from build123d import *

# Parameters (mm, degrees)
F0_W            = 50
F0_H            = 150
F0_H_2          = 50
F0_W_2          = 60
F0_W_3          = 70
F0_H_3          = 35
F1_DEPTH        = 10
F2_W            = 10
F2_H            = 50
F3_DEPTH        = 30
F4_R            = 5.5
F5_DEPTH        = 190.001
F6_R            = 3.175
F7_DEPTH        = 10.001
F8_R            = 5.5
F9_DEPTH        = 10.001
F10_R           = 5.5
F11_DEPTH       = 10.001
F13_DEPTH       = 10.001
F14_W           = 6
F14_H           = 30
F15_DEPTH       = 32
F16_R           = 5.5
F17_DEPTH       = 76.001
F19_D           = 3.1
F19_CSINK_D     = 5.6
F19_CSINK_ANGLE = 90
F21_D           = 2
F21_DEPTH       = 30
F21_TIP         = 0.600860619


with BuildPart() as f1:
    # F0 (on Top) → F1 (new body)
    with BuildSketch(Plane.XY):
        Rectangle(F0_W, F0_H)
        with Locations((0, 100)):
            Rectangle(F0_W, F0_H_2)
        with Locations((55, 100)):
            Rectangle(F0_W_2, F0_H_2)
        with Locations((-55, 100)):
            Rectangle(F0_W_2, F0_H_2)
        with Locations((0, -100)):
            Rectangle(F0_W, F0_H_2)
        with Locations((60, -100)):
            Rectangle(F0_W_3, F0_H_2)
        with Locations((0, 142.5)):
            Rectangle(F0_W, F0_H_3)
        with Locations((-60, -100)):
            Rectangle(F0_W_3, F0_H_2)
    extrude(amount=F1_DEPTH)

    # F2 (on face) → F3 (join)
    with BuildSketch(Plane.XY.offset(10)):
        with Locations((-90, -100)):
            Rectangle(F2_W, F2_H)
        with Locations((90, -100)):
            Rectangle(F2_W, F2_H)
    extrude(amount=F3_DEPTH)

    # F4 (on face) → F5 (cut, through all)
    with BuildSketch(Plane(origin=(-95, 0, 0), x_dir=(0, -1, 0), z_dir=(-1, 0, 0))):
        with Locations((100, 30.5)):
            Circle(F4_R)
    extrude(amount=-F5_DEPTH, mode=Mode.SUBTRACT)

    # F6 (on face) → F7 (cut, through all)
    with BuildSketch(Plane.XY.offset(10)):
        with Locations((0, 152.825)):
            Circle(F6_R)
    extrude(amount=-F7_DEPTH, mode=Mode.SUBTRACT)

    # F8 (on face) → F9 (cut, through all)
    with BuildSketch(Plane.XY.offset(10)):
        with Locations((-69.5, 100)):
            Circle(F8_R)
    extrude(amount=-F9_DEPTH, mode=Mode.SUBTRACT)

    # F10 (on face) → F11 (cut, through all)
    with BuildSketch(Plane.XY.offset(10)):
        with Locations((69.5, 100)):
            Circle(F10_R)
    extrude(amount=-F11_DEPTH, mode=Mode.SUBTRACT)

    # F12 (on face) → F13 (cut, through all)
    with BuildSketch(Plane.XY.offset(10)):
        with BuildLine():
            Line((17.7911710483, 82.2515942001), (27.4237727452, 85))
            ThreePointArc((27.4237727452, 85), (24.83, 100), (27.4237727452, 115))
            Line((27.4237727452, 115), (17.7911710483, 117.7484057999))
            ThreePointArc((17.7911710483, 117.7484057999), (14.83, 100), (17.7911710483, 82.2515942001))
        make_face()
        with BuildLine():
            Line((-27.4237727452, 85), (-17.7911710483, 82.2515942001))
            ThreePointArc((-17.7911710483, 82.2515942001), (-14.83, 100), (-17.7911710483, 117.7484057999))
            Line((-17.7911710483, 117.7484057999), (-27.4237727452, 115))
            ThreePointArc((-27.4237727452, 115), (-24.83, 100), (-27.4237727452, 85))
        make_face()
    extrude(amount=-F13_DEPTH, mode=Mode.SUBTRACT)

    # F14 (on face) → F15 (join)
    with BuildSketch(Plane.XY.offset(10)):
        with Locations((22, 6.836565081)):
            Rectangle(F14_W, F14_H)
    extrude(amount=F15_DEPTH)

    # F16 (on face) → F17 (cut, through all)
    with BuildSketch(Plane(origin=(19, 0, 0), x_dir=(0, -1, 0), z_dir=(-1, 0, 0))):
        with Locations((-6.426565081, 30.5)):
            Circle(F16_R)
    extrude(amount=-F17_DEPTH, mode=Mode.SUBTRACT)

    # F19 (through all)
    with Locations(Plane.YZ.offset(25)):
        with Locations((6.426565081, 38.4), (14.326565081, 30.5), (6.426565081, 22.6), (-1.473434919, 30.5)):
            CounterSinkHole(F19_D / 2, F19_CSINK_D / 2, counter_sink_angle=F19_CSINK_ANGLE)

    # F21
    with Locations(Plane.YZ.offset(95)):
        with Locations((-107.1, 30.5), (-92.9, 30.5), (-91.0878232998, 21.4521767002), (-109.0478232998, 21.5878232998)):
            Hole(F21_D / 2, depth=F21_DEPTH)
            with Locations((0, 0, -(F21_DEPTH + F21_TIP / 2))):  # 118° drill point
                Cone(0, F21_D / 2, F21_TIP, mode=Mode.SUBTRACT)


solid = f1.part
For this review, take the finished solid that the model builds, in its own axes (mm). A direction names the side the tool comes from. Give positions to 0.01 mm unless a question says otherwise; leave off trailing zeros. Loops run counter-clockwise (first coordinate to the right, second up) from the corner with the lowest first, then second, coordinate; pieces in that order, holes last. Notation, with made-up numbers: M 43.5,88 L 90.5,88 A9 ccw 90.5,102 Z; hole C 89,-10.5 d5. An arc over 180 degrees is marked long. Answer as a JSON object with one key per item and string values. Group by question number.
Q1. For probe 1 along Y at (x, z) = (20.15, 30.5); probe 2 along Y at (x, z) = (-69.5, 5); probe 3 along Y at (x, z) = (0, 6.5), list the stretches that pass through material, from the lowest coordinate up. Write a range as [from, to].
Q2. Mouldability with a two-part tool opening along Y and no side actions: class faces 1 (the cylindrical face through (-90.07, -94.505, 30.742)), 2 (the flat face through (22, -8.163, 26)), 3 (the flat face through (22, 7, 42)), 4 (the cylindrical face through (-14.83, 99.75, 5.07)) as +Y half, -Y half, draft (parallel to the pull), parting line (faces both ways), or undercut.
Q3. Add section D-D on y = 100. Give the boundary of the cut face in (x, z).
Q4. Insertion check: P1, Ø3, axis at x = 23, z = 21, coming from the +Y side; P2, Ø10, axis at x = 0.5, y = -67, coming from the +Z side; P3, Ø6.5, axis at y = 6.43, z = 30.5, coming from the -X side; P4, Ø4, axis at y = 21, z = 8.5, coming from the +X side. Each pin has a flat end and moves straight along its axis. Give the tip position at first contact, or say it passes through.
Q5. Tool access review of faces 5 (the flat face through (-67.9, -75, 9.5)), 6 (the flat face through (-85, -100.4, 24.8)), 7 (the flat face through (70, -75, 8)), 8 (the cylindrical face through (14.83, 100.25, 5.07)), 9 (the flat face through (55, 125, 5)): name each direction out of +Z, -Z, +X, -X, +Y, -Y from which nothing blocks a thin tool from reaching the whole face with its end or side.
Q6. Add section C-C on z = 16. Give the boundary of the cut face in (x, y).
Q7. Add section B-B on y = -100. Give the boundary of the cut face in (x, z).
Q8. Add section A-A on x = 0. Give the boundary of the cut face in (y, z).
Checked values:
{
 "1": {"probe 1": "[-8.16, -3.02], [0.08, 0.93], [11.93, 12.78], [15.88, 21.84]", "probe 2": "[-125, -75], [75, 94.5], [105.5, 125]", "probe 3": "[-125, 149.65], [156, 160]"},
 "2": {"face 1": "undercut", "face 2": "-Y half", "face 3": "draft", "face 4": "undercut"},
 "3": {"outline": "M -85,0 L -75,0 L -75,10 L -85,10 Z; M -64,0 L -24.83,0 L -24.83,10 L -64,10 Z; M -14.83,0 L 14.83,0 L 14.83,10 L -14.83,10 Z; M 24.83,0 L 64,0 L 64,10 L 24.83,10 Z; M 75,0 L 85,0 L 85,10 L 75,10 Z"},
 "4": {"P1": "y = 21.84", "P2": "z = 10", "P3": "through", "P4": "x = 25"},
 "5": {"face 5": "+Z, -Z, -X", "face 6": "+Z, +Y, -Y", "face 7": "+Z, -Z, +X", "face 8": "+Z, -Z", "face 9": "+Z, -Z, +X, +Y"},
 "6": {"outline": "M -95,-125 L -85,-125 L -85,-75 L -95,-75 Z; M 19,-8.16 L 25,-8.16 L 25,21.84 L 19,21.84 Z; M 85,-125 L 95,-125 L 95,-75 L 85,-75 Z"},
 "7": {"outline": "M -95,0 L 95,0 L 95,25 L 85,25 L 85,10 L -85,10 L -85,25 L -95,25 Z; M -95,36 L -85,36 L -85,40 L -95,40 Z; M 85,36 L 95,36 L 95,40 L 85,40 Z"},
 "8": {"outline": "M -125,0 L 149.65,0 L 149.65,10 L -125,10 Z; M 156,0 L 160,0 L 160,10 L 156,10 Z"}
}
